Could you check a few things on this drawing? It's one solid part, dimensions in mm from its lowest x, y, z. A direction names the side the tool comes from. Coordinates: 2 decimals unless noted, no trailing zeros. Loops run counter-clockwise (first coordinate to the right, second up) from the corner with the lowest first, then second, coordinate; pieces in that order, holes last. Notation, with made-up numbers: M 63.5,-34.75 L 95.5,-34.75 A25 ccw 95.5,-0.75 Z; hole C 29.5,15.25 d6. An arc over 180 degrees is marked long. Use one line per item in the form item = value. Start each with the question number.
(1) Imagine slicing it at A-A, the plane y = 4.5. Please give me the cut outline in (x, z).
(2) Imagine slicing it at C-C, the plane x = 15.5. Please give me the cut outline in (y, z).
(3) Will these pins go through, and if not, where does the flat tip stop? P1, Ø0.8, axis at y = 1.5, z = 4, coming from the +X side; P2, Ø1.8, axis at x = 0.5, z = 3, coming from the +Y side; P3, Ø3, axis at x = 10, z = 4.5, coming from the -Y side.
(4) Please list where these lines run through material, in increasing order: L1, parallel to Y at x = 4.5, z = 2.8; L2, parallel to X at y = 4.5, z = 3; L3, parallel to Z at x = 15, y = 4.
(5) On a 3-axis mill with a long thin cutter (end or side, diameter ignored), from which of +Z, -Z, +X, -X, +Y, -Y can I reach the whole of each face in a straight line? I mean the marked faces 1, 2 and 3. Say none if no direction works.
(6) Imagine slicing it at B-B, the plane x = 4.5. Please give me the cut outline in (y, z).
(7) Imagine slicing it at D-D, the plane x = 9.5. Please give me the cut outline in (y, z).
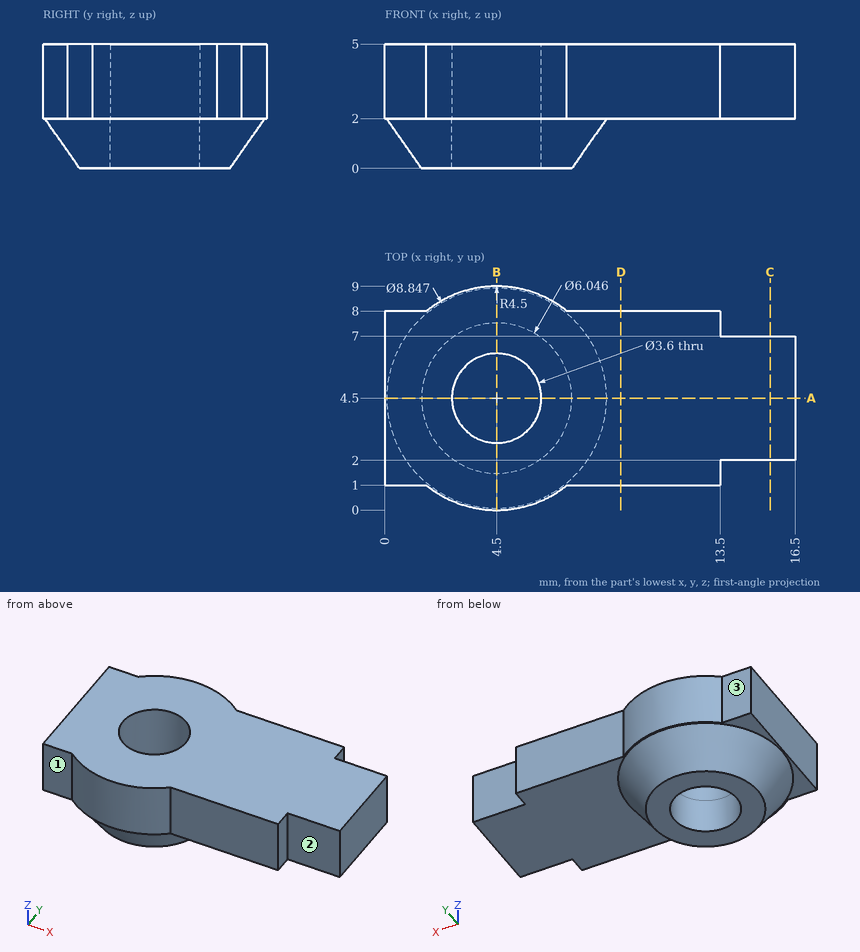
Answer:
q1.outline = M 0,2 L 0.08,2 L 1.48,0 L 2.7,0 L 2.7,5 L 0,5 Z; M 6.3,0 L 7.52,0 L 8.92,2 L 16.5,2 L 16.5,5 L 6.3,5 Z
q2.outline = M 2,2 L 7,2 L 7,5 L 2,5 Z
q3.P1 = 13.5
q3.P2 = 8
q3.P3 = 1
q4.L1 = 0 to 2.7, 6.3 to 9
q4.L2 = 0 to 2.7, 6.3 to 16.5
q4.L3 = 2 to 5
q5.face_1 = +Z, -Z, -X, -Y
q5.face_2 = +Z, -Z, +X, -Y
q5.face_3 = +Z, -Z, -X, +Y
q6.outline = M 0,2 L 0.08,2 L 1.48,0 L 2.7,0 L 2.7,5 L 0,5 Z; M 6.3,0 L 7.52,0 L 8.92,2 L 9,2 L 9,5 L 6.3,5 Z
q7.outline = M 1,2 L 8,2 L 8,5 L 1,5 Z
